from build123d import *

# Parameters (mm, degrees)
BOSS_EXTRUDE1_DEPTH = 3
SKETCH2_R           = 2.05
CUT_EXTRUDE1_DEPTH  = 45.877826774
LPATTERN1_COUNT     = 5
LPATTERN1_PITCH     = 8
SKETCH3_R           = 2.05
CUT_EXTRUDE2_DEPTH  = 45.877826774
LPATTERN2_COUNT     = 5
LPATTERN2_PITCH     = 8


with BuildPart() as part:
    # Sketch1 → Boss-Extrude1 (new body)
    with BuildSketch(Plane.XY):
        with BuildLine():
            Line((3.313708499, 4), (32, 4))
            ThreePointArc((32, 4), (36, 0), (32, -4))
            Line((32, -4), (0, -4))
            ThreePointArc((0, -4), (-1.530733729, -3.69551813), (-2.828427125, -2.828427125))
            Line((-2.828427125, -2.828427125), (-25.455844123, 19.798989873))
            ThreePointArc((-25.455844123, 19.798989873), (-25.455844123, 25.455844123), (-19.798989873, 25.455844123))
            Line((-19.798989873, 25.455844123), (0.485281374, 5.171572875))
            ThreePointArc((0.485281374, 5.171572875), (1.78297477, 4.30448187), (3.313708499, 4))
        make_face()
    extrude(amount=BOSS_EXTRUDE1_DEPTH)

    # Sketch2 → Cut-Extrude1 (cut, through all)
    with BuildSketch(Plane.XY.offset(3)):
        with Locations((-22.627416998, 22.627416998)):
            Circle(SKETCH2_R)
    cut_extrude1 = extrude(amount=-CUT_EXTRUDE1_DEPTH, mode=Mode.SUBTRACT)

    # LPattern1: Cut-Extrude1 ×5
    with Locations(*[Vector(0.7071067811865515, -0.7071067811865437, 0) * (i * LPATTERN1_PITCH) for i in range(1, LPATTERN1_COUNT)]):
        add(cut_extrude1, mode=Mode.SUBTRACT)

    # Sketch3 → Cut-Extrude2 (cut, through all)
    with BuildSketch(Plane.XY.offset(3)):
        with Locations((32, 0)):
            Circle(SKETCH3_R)
    cut_extrude2 = extrude(amount=-CUT_EXTRUDE2_DEPTH, mode=Mode.SUBTRACT)

    # LPattern2: Cut-Extrude2 ×5
    with Locations(*[(-i * LPATTERN2_PITCH, 0, 0) for i in range(1, LPATTERN2_COUNT)]):
        add(cut_extrude2, mode=Mode.SUBTRACT)


solid = part.part
Read the model definition and answer for the solid it produces. Units are mm, in the model's axes. A direction names the side the tool comes from. Round coordinates to 2 decimals unless told otherwise and drop trailing zeros. Loops run counter-clockwise (first coordinate to the right, second up) from the corner with the lowest first, then second, coordinate; pieces in that order, holes last.
Q1. Consider probe 1 along Y at (x, z) = (8, 1.7); probe 2 along X at (y, z) = (1, 1); probe 3 along Y at (x, z) = (0, 1.7). Determine where each line is inside the solid, lowest interval first.
Q2. Determine the mould class of faces 3 (the face through (36, 0, 1)), 4 (the face through (-13.984, 8.327, 1.479)), 5 (the face through (-20.734, 21.842, 1.521)) for opening direction Y: released by +Y, released by -Y, zero draft, split by the parting line, or undercut.
Q3. Which of the six approach directions +Z, -Z, +X, -X, +Y, -Y give full straight-line access (tool end or side, diameter ignored) to faces 1 (the face through (13.95, 0.09, 1.52)), 2 (the face through (17, 4, 1))?
Q4. Section C-C on y = 24 is taken. Write down the section's boundary in (x, z).
Q5. Section A-A on x = 16 is taken. Write down the section's boundary in (y, z), and give its area (3 significant figures).
Q6. Each of these flat-tipped pins is pushed along its axis until it touches: pin 1 (1.5 mm diameter, centred on y = 5.5, z = 0.5, fed in from -X); pin 2 (0.9 mm diameter, centred on x = 19.5, z = 1, fed in from +Y). Where does it stop, or does it pass through?
Q7. Section B-B on y = -1 is taken. Write down the section's boundary in (x, z).
Q8. Section D-D on z = 0.8 is taken. Give the number of separate pieces and of enclosed holes in the cut face, and give its area (3 significant figures).
Output:
1. probe 1: y = -4 to -2.05, 2.05 to 4
1. probe 2: x = -6.66 to -1.79, 1.79 to 6.21, 9.79 to 14.21, 17.79 to 22.21, 25.79 to 30.21, 33.79 to 35.87
1. probe 3: y = -4 to -2.05, 2.05 to 5.66
2. face 3: split by the parting line
2. face 4: released by -Y
2. face 5: undercut
3. face 1: +Z, -Z
3. face 2: +Z, -Z, +X, +Y
4. outline: (-26.38, 0) - (-24.15, 0) - (-24.15, 3) - (-26.38, 3) - close; (-21.1, 0) - (-18.34, 0) - (-18.34, 3) - (-21.1, 3) - close
5. outline: (-4, 0) - (-2.05, 0) - (-2.05, 3) - (-4, 3) - close; (2.05, 0) - (4, 0) - (4, 3) - (2.05, 3) - close
5. area: 11.7 mm2
6. pin 1: stops at x = -11.91
6. pin 2: stops at y = 4
7. outline: (-4.66, 0) - (-1.79, 0) - (-1.79, 3) - (-4.66, 3) - close; (1.79, 0) - (6.21, 0) - (6.21, 3) - (1.79, 3) - close; (9.79, 0) - (14.21, 0) - (14.21, 3) - (9.79, 3) - close; (17.79, 0) - (22.21, 0) - (22.21, 3) - (17.79, 3) - close; (25.79, 0) - (30.21, 0) - (30.21, 3) - (25.79, 3) - close; (33.79, 0) - (35.87, 0) - (35.87, 3) - (33.79, 3) - close
8. separate pieces: 1
8. enclosed holes: 9
8. area: 443 mm2
